from build123d import *

# Parameters (mm, degrees)
ESQUISSE1_R        = 20
BOSS_EXTRU_1_DEPTH = 4
ESQUISSE2_R        = 2.5
BOSS_EXTRU_2_DEPTH = 7.5
ESQUISSE3_R        = 0.966516747
BOSS_EXTRU_3_DEPTH = 2
ESQUISSE4_R        = 1.5
BOSS_EXTRU_4_DEPTH = 7.5


with BuildPart() as part:
    # Esquisse1 → Boss.-Extru.1 (new body)
    with BuildSketch(Plane.XY):
        Circle(ESQUISSE1_R)
        with BuildLine():
            Line((-15.874507866, 2), (-2, 2))
            Line((-2, 2), (-2, 15.874507866))
            ThreePointArc((-2, 15.874507866), (-11.313708499, 11.313708499), (-15.874507866, 2))
        make_face(mode=Mode.SUBTRACT)
        with BuildLine():
            Line((-15.874507866, -2), (-2, -2))
            Line((-2, -2), (-2, -15.874507866))
            ThreePointArc((-2, -15.874507866), (-11.313708499, -11.313708499), (-15.874507866, -2))
        make_face(mode=Mode.SUBTRACT)
        with BuildLine():
            Line((2, 15.874507866), (2, 2))
            Line((2, 2), (15.874507866, 2))
            ThreePointArc((15.874507866, 2), (11.313708499, 11.313708499), (2, 15.874507866))
        make_face(mode=Mode.SUBTRACT)
        with BuildLine():
            Line((2, -2), (2, -15.874507866))
            ThreePointArc((2, -15.874507866), (11.313708499, -11.313708499), (15.874507866, -2))
            Line((15.874507866, -2), (2, -2))
        make_face(mode=Mode.SUBTRACT)
    extrude(amount=BOSS_EXTRU_1_DEPTH)

    # Esquisse2 → Boss.-Extru.2 (add, symmetric)
    with BuildSketch(Plane.XY.offset(4)):
        Circle(ESQUISSE2_R)
    extrude(amount=BOSS_EXTRU_2_DEPTH, both=True)

    # Esquisse3 → Boss.-Extru.3 (add)
    with BuildSketch(Plane.XY.offset(11.5)):
        Circle(ESQUISSE3_R)
    extrude(amount=BOSS_EXTRU_3_DEPTH)

    # Esquisse4 → Boss.-Extru.4 (add)
    with BuildSketch(Plane.XY.offset(4)):
        with Locations((8, 0)):
            Circle(ESQUISSE4_R)
        with Locations((-8, 0)):
            Circle(ESQUISSE4_R)
    extrude(amount=BOSS_EXTRU_4_DEPTH)


solid = part.part
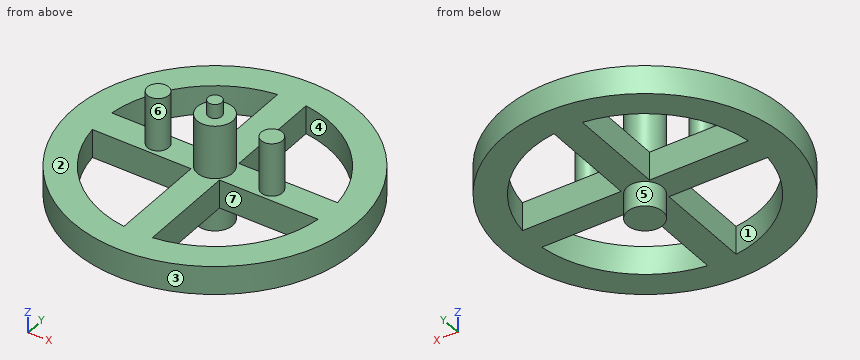
Design review of the part built by this model. Coordinates are the model's own, in mm. Face numbers are marked on the shaded views. A direction names the side the tool comes from. Round coordinates to 2 decimals unless told otherwise and drop trailing zeros. Write each loop counter-clockwise with the first axis right and the second up, starting at its lowest first coordinate (ties: lowest second). Pieces come first, ordered by that corner, then holes. Notation, with made-up numbers: M -14,72.5 L 9,72.5 A25 cw 9,95.5 Z; hole C 48,35 d8. An arc over 180 degrees is marked long. One line per item, written item: value. Start each with the question number.
1. Draft analysis for pull direction Y (two halves, no side actions). For the marked faces 1, 2, 3 and 4, state which applies: pulls with the +Y half, pulls with the -Y half, needs draft (parallel to the pull), parting line crosses it, or undercut.
2. Take a section at B-B on z = 3.5. State the section outline as (x, y) points.
3. Take a section at D-D on y = -11. State the section outline as (x, z) points.
4. To check wall thickness, follow probe 1 along Y at (x, z) = (-6, 1.5); probe 2 along X at (y, z) = (-9.5, 3.5); probe 3 along X at (y, z) = (10, 2.5). State the ranges of each line that lie inside material, in increasing order. Write a range as from..to.
5. For the marked faces 5, 6 and 7, list the 3-axis set-ups (+Z, -Z, +X, -X, +Y, -Y) from which the entire face can be reached by the end or side of a thin tool; tool diameter is ignored.
6. Take a section at C-C on z = 6.5. State the section outline as (x, y) points.
7. Clearance check with flat-ended pins moving along their axes: P1, Ø2, axis at y = 13, z = -0.5, coming from the +X side; P2, Ø1, axis at x = 8, z = 3, coming from the +Y side; P3, Ø1.2, axis at x = 8, z = 2.5, coming from the -Y side; P4, Ø1.5, axis at x = -5, y = 12.5, coming from the -Z side (3 decimals). State where each tip first meets the part, or that it passes through.
8. Take a section at A-A on x = 10. State the section outline as (y, z) points.
Computed:
1. face 1: undercut
1. face 2: needs draft
1. face 3: parting line crosses it
1. face 4: undercut
2. outline: C 0,0 d40; hole M -15.87,-2 A16 ccw -2,-15.87 L -2,-2 Z; hole M -15.87,2 L -2,2 L -2,15.87 A16 ccw Z; hole M 2,-15.87 A16 ccw 15.87,-2 L 2,-2 Z; hole M 2,2 L 15.87,2 A16 ccw 2,15.87 Z
3. outline: M -16.7,0 L -11.62,0 L -11.62,4 L -16.7,4 Z; M -2,0 L 2,0 L 2,4 L -2,4 Z; M 11.62,0 L 16.7,0 L 16.7,4 L 11.62,4 Z
4. probe 1: y = -19.08..-14.83, -2..2, 14.83..19.08
4. probe 2: x = -17.6..-12.87, -2..2, 12.87..17.6
4. probe 3: x = -17.32..-12.49, -2..2, 12.49..17.32
5. face 5: -Z
5. face 6: +Z
5. face 7: +Z, -Z
6. outline: C -8,0 d3; C 0,0 d5; C 8,0 d3
7. P1: stops at x = 15.9
7. P2: stops at y = 18.54
7. P3: stops at y = -18.58
7. P4: passes through
8. outline: M -17.32,0 L -12.49,0 L -12.49,4 L -17.32,4 Z; M -2,0 L 2,0 L 2,4 L -2,4 Z; M 12.49,0 L 17.32,0 L 17.32,4 L 12.49,4 Z
